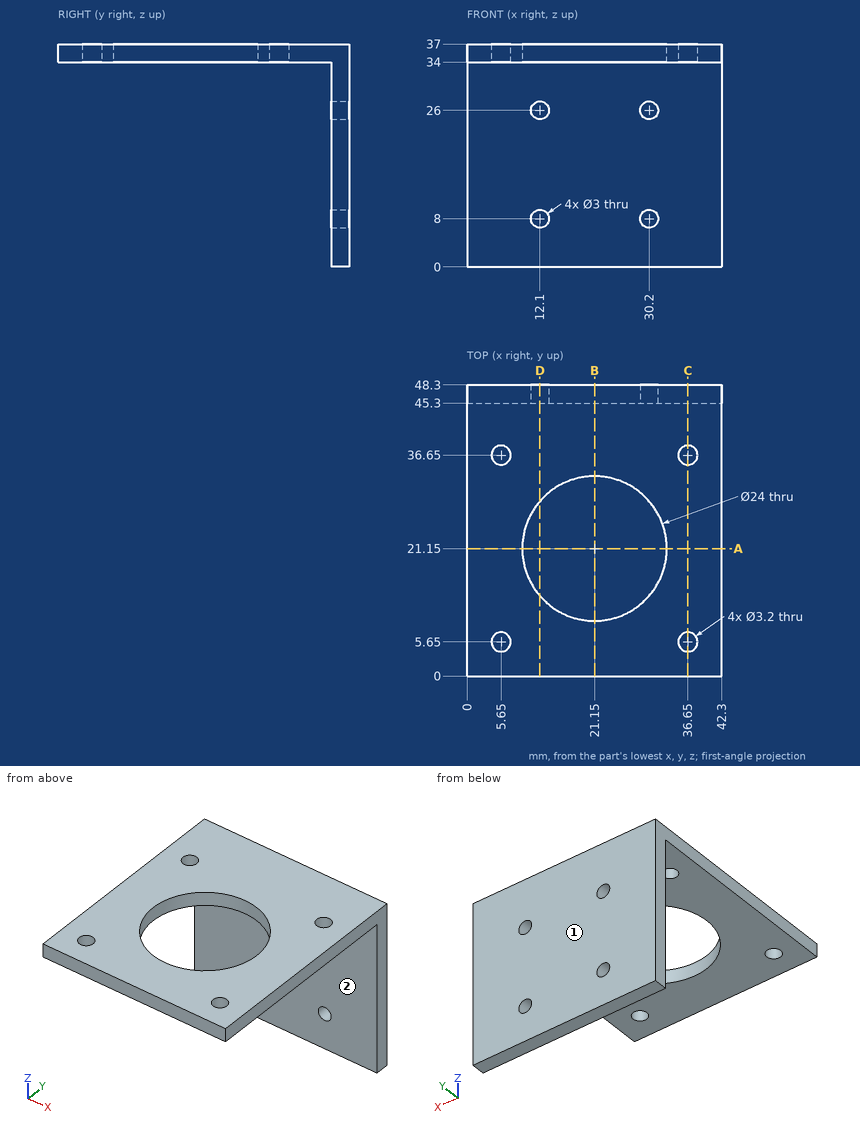
Source: three-view drawing plus pictorial views. Frame: mm from the lowest corner of the part. A direction names the side the tool comes from. Give positions to 0.01 mm unless a question says otherwise; leave off trailing zeros. Order: outer loops, then holes, each group sorted by start corner. A loop starts at its lowest first (then second) coordinate and runs counter-clockwise, first axis right, second up. Notation, with made-up numbers: (9, 48) - (15, 48) arc R24 ccw to (15, 58) - close; hole circle Ø1 at (-10, 22). An arc over 180 degrees is marked (long way). Put each result on its own line as item: value.
Item 1: Contact query for flat-ended pins moving along their axis: pin 1 (3.5 mm diameter, centred on x = 30.2, z = 26, fed in from +Y); pin 2 (10 mm diameter, centred on x = 11.5, z = 19, fed in from -Y); pin 3 (1.5 mm diameter, centred on x = 5, y = 8.5, fed in from -Z). Output: stop coordinate, or through.
Found:
pin 1: stops at y = 48.3
pin 2: stops at y = 45.3
pin 3: stops at z = 34
Item 2: Section query C-C, the plane x = 36.65. Return loops of the section in (y, z).
Found:
outline: (0, 34) - (4.05, 34) - (4.05, 37) - (0, 37) - close; (7.25, 34) - (35.05, 34) - (35.05, 37) - (7.25, 37) - close; (38.25, 34) - (45.3, 34) - (45.3, 0) - (48.3, 0) - (48.3, 37) - (38.25, 37) - close
Item 3: Section query D-D, the plane x = 12.1. Return loops of the section in (y, z), then the cut area to 3 significant figures.
Found:
outline: (0, 34) - (13.27, 34) - (13.27, 37) - (0, 37) - close; (29.03, 34) - (45.3, 34) - (45.3, 27.5) - (48.3, 27.5) - (48.3, 37) - (29.03, 37) - close; (45.3, 0) - (48.3, 0) - (48.3, 6.5) - (45.3, 6.5) - close; (45.3, 9.5) - (48.3, 9.5) - (48.3, 24.5) - (45.3, 24.5) - close
area: 182 mm^2
Item 4: Access query for the marked faces 1 and 2. Directions: +Z, -Z, +X, -X, +Y, -Y. A direction counts if a zero-diameter tool reaches every point of the face in a straight line with its end or side. Return the directions, or none.
Found:
face 1: +Z, -Z, +X, -X, +Y
face 2: -Z, +X, -X, -Y
Item 5: Section query A-A, the plane y = 21.15. Return loops of the section in (x, z).
Found:
outline: (0, 34) - (9.15, 34) - (9.15, 37) - (0, 37) - close; (33.15, 34) - (42.3, 34) - (42.3, 37) - (33.15, 37) - close
Item 6: Ray query, L1, parallel to Z at x = 30.2, y = 46.2; L2, parallel to Y at x = 5.65, z = 35.85; L3, parallel to Y at x = 31.5, z = 21. Return the intervals inside material, ascending. Write a range as from..to.
Found:
L1: z = 0..6.5, 9.5..24.5, 27.5..37
L2: y = 0..4.05, 7.25..35.05, 38.25..48.3
L3: y = 45.3..48.3
Item 7: Section query B-B, the plane x = 21.15. Return loops of the section in (y, z).
Found:
outline: (0, 34) - (9.15, 34) - (9.15, 37) - (0, 37) - close; (33.15, 34) - (45.3, 34) - (45.3, 0) - (48.3, 0) - (48.3, 37) - (33.15, 37) - close
